Source: CAD feature listing. Evaluate the final solid. Frame: model axes, mm. A direction names the side the tool comes from. Coordinates: 2 decimals unless noted, no trailing zeros. Order: outer loops, then holes, each group sorted by start corner. A loop starts at its lowest first (then second) coordinate and runs counter-clockwise, first axis right, second up.
Item 1: Mould query, pull axis Y, two halves, no side actions, for faces 1 (the cylindrical face through (89.505, -20.242, 3.796)), 2 (the flat face through (95.2, -10.8, 15)), 3 (the flat face through (54.2, -40, 25.7)), 4 (the cylindrical face through (20.246, -21.652, 3.796)). Classes: released by +Y, released by -Y, zero draft, split by the parting line, or undercut.
Item 2: Section D-D on z = 9. Return the cut outline in (x, y), then the cut area to 3 significant figures.
Item 3: Section A-A on y = -20. Return the cut outline in (x, z).
Item 4: Section B-B on x = 15. Return the cut outline in (y, z).
Item 5: Ray query, line 1 (X direction, y = -20, z = 5); line 2 (Y direction, x = 95, z = 12); line 3 (Y direction, x = 95, z = 5.25). Return the intervals inside material, ascending.
Item 6: Section C-C on y = -3. Return the cut outline in (x, z).
Item 7: Reachability of faces 5 (the flat face through (30, -20, 28)), 6 (the flat face through (91, -24, 7.7)), 7 (the flat face through (80, -20, 27)) from +Z, -Z, +X, -X, +Y, -Y: full face, straight path, thin tool, end or side. Return the list, or none.
Item 8: Contact query for flat-ended pins moving along their axis: P1, Ø7.5, axis at y = -12, z = 22.5, coming from the +X side; P2, Ø7.5, axis at y = -24, z = 32, coming from the -X side; P3, Ø2, axis at x = 49.5, y = -31.5, coming from the +Z side. Output: stop coordinate, or through.
from build123d import *

# Parameters (mm, degrees)
F1_DEPTH = 40
F2_R     = 9
F3_DEPTH = 7.3
F4_R     = 5.5
F5_DEPTH = 7.7
F6_R     = 9
F7_DEPTH = 7.3


with BuildPart() as f1:
    # F0 (on Front) → F1 (new body)
    with BuildSketch(Plane.XZ):
        with BuildLine():
            Line((0, 15), (0, 0))
            Line((0, 0), (55, 0))
            Line((55, 0), (55, 26))
            ThreePointArc((55, 26), (41, 40), (55, 54))
            Line((55, 54), (55, 65))
            ThreePointArc((55, 65), (37.3223304703, 57.6776695297), (30, 40))
            Line((30, 40), (30, 15))
            Line((30, 15), (0, 15))
        make_face()
        with BuildLine():
            Line((55, 26), (55, 0))
            Line((55, 0), (110, 0))
            Line((110, 0), (110, 15))
            Line((110, 15), (80, 15))
            Line((80, 15), (80, 40))
            ThreePointArc((80, 40), (72.6776695297, 57.6776695297), (55, 65))
            Line((55, 65), (55, 54))
            ThreePointArc((55, 54), (64.8994949366, 49.8994949366), (69, 40))
            ThreePointArc((69, 40), (64.8994949366, 30.1005050634), (55, 26))
        make_face()
    extrude(amount=F1_DEPTH)

    # F2 (on face) → F3 (cut)
    with BuildSketch(Plane.XY.offset(15)):
        with Locations((15, -20)):
            Circle(F2_R)
    extrude(amount=-F3_DEPTH, mode=Mode.SUBTRACT)

    # F4 (on face) → F5 (cut)
    with BuildSketch(Plane(origin=(0, 0, 0), x_dir=(1, 0, 0), z_dir=(0, 0, -1))):
        with Locations((15, 20)):
            Circle(F4_R)
        with Locations((95, 20)):
            Circle(F4_R)
    extrude(amount=-F5_DEPTH, mode=Mode.SUBTRACT)

    # F6 (on face) → F7 (cut)
    with BuildSketch(Plane.XY.offset(15)):
        with Locations((95, -20)):
            Circle(F6_R)
    extrude(amount=-F7_DEPTH, mode=Mode.SUBTRACT)


solid = f1.part
Answer list:
1. face 1: undercut
1. face 2: zero draft
1. face 3: released by -Y
1. face 4: undercut
2. outline: (0, -40) - (110, -40) - (110, 0) - (0, 0) - close; hole circle Ø18 at (15, -20); hole circle Ø18 at (95, -20)
2. area: 3,890 mm2
3. outline: (0, 0) - (9.5, 0) - (9.5, 7.7) - (6, 7.7) - (6, 15) - (0, 15) - close; (20.5, 0) - (89.5, 0) - (89.5, 7.7) - (86, 7.7) - (86, 15) - (80, 15) - (80, 40) arc R25 ccw to (30, 40) - (30, 15) - (24, 15) - (24, 7.7) - (20.5, 7.7) - close; (100.5, 0) - (110, 0) - (110, 15) - (104, 15) - (104, 7.7) - (100.5, 7.7) - close; hole circle Ø28 at (55, 40)
4. outline: (-40, 0) - (-25.5, 0) - (-25.5, 7.7) - (-29, 7.7) - (-29, 15) - (-40, 15) - close; (-14.5, 0) - (0, 0) - (0, 15) - (-11, 15) - (-11, 7.7) - (-14.5, 7.7) - close
5. line 1: x = 0 to 9.5, 20.5 to 89.5, 100.5 to 110
5. line 2: y = -40 to -29, -11 to 0
5. line 3: y = -40 to -25.5, -14.5 to 0
6. outline: (0, 0) - (110, 0) - (110, 15) - (80, 15) - (80, 40) arc R25 ccw to (30, 40) - (30, 15) - (0, 15) - close; hole circle Ø28 at (55, 40)
7. face 5: +Z, -X, +Y, -Y
7. face 6: +Z
7. face 7: +Z, +X, +Y, -Y
8. P1: stops at x = 80
8. P2: stops at x = 30
8. P3: stops at z = 64.59
